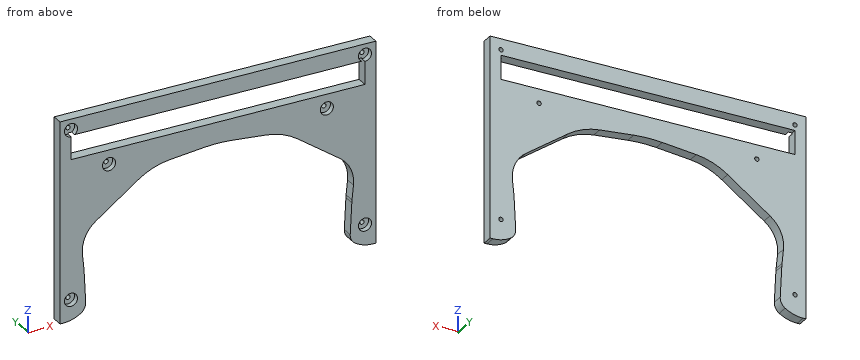
```python
from build123d import *

# Parameters (mm, degrees)
BOSS_EXTRU_1_DEPTH       = 10
ESQUISSE3_R              = 2
ENL_V_MAT_EXTRU_1_DEPTH  = 10
ESQUISSE6_W              = 270
ESQUISSE6_H              = 22
ENL_V_MAT_EXTRU_4_DEPTH  = 10
ESQUISSE9_R              = 2
ENL_V_MAT_EXTRU_7_DEPTH  = 10
ENL_V_MAT_EXTRU_9_DEPTH  = 10
CONG_5_R                 = 10
ESQUISSE12_R             = 2
ENL_V_MAT_EXTRU_10_DEPTH = 10
ESQUISSE14_R             = 6
ENL_V_MAT_EXTRU_11_DEPTH = 5


with BuildPart() as part:
    # Esquisse2 → Boss.-Extru.1 (new body)
    with BuildSketch(Plane(origin=(0, 0, 0), x_dir=(1, 0, 0), z_dir=(0, 1, 0))):
        with BuildLine():
            Line((0, 0), (290, 0))
            Line((290, 0), (290, 184.53))
            Line((290, 184.53), (287.426406871, 184.53))
            ThreePointArc((287.426406871, 184.53), (275.9459039, 182.246385975), (266.213203436, 175.743203436))
            Line((266.213203436, 175.743203436), (180.47, 90))
            Line((180.47, 90), (109.53, 90))
            Line((109.53, 90), (23.786796564, 175.743203436))
            ThreePointArc((23.786796564, 175.743203436), (14.0540961, 182.246385975), (2.573593129, 184.53))
            Line((2.573593129, 184.53), (0, 184.53))
            Line((0, 184.53), (0, 0))
        make_face()
    extrude(amount=BOSS_EXTRU_1_DEPTH)

    # Esquisse3 → Enlèv. mat.-Extru.1 (cut)
    with BuildSketch(Plane(origin=(0, 10, 0), x_dir=(1, 0, 0), z_dir=(0, 1, 0))):
        with Locations((10, 10)):
            Circle(ESQUISSE3_R)
        with Locations((280, 10)):
            Circle(ESQUISSE3_R)
    extrude(amount=-ENL_V_MAT_EXTRU_1_DEPTH, mode=Mode.SUBTRACT)

    # Esquisse6 → Enlèv. mat.-Extru.4 (cut)
    with BuildSketch(Plane(origin=(0, 10, 0), x_dir=(1, 0, 0), z_dir=(0, 1, 0))):
        with Locations((145, 26)):
            Rectangle(ESQUISSE6_W, ESQUISSE6_H)
    extrude(amount=-ENL_V_MAT_EXTRU_4_DEPTH, mode=Mode.SUBTRACT)

    # Esquisse9 → Enlèv. mat.-Extru.7 (cut)
    with BuildSketch(Plane(origin=(0, 10, 0), x_dir=(1, 0, 0), z_dir=(0, 1, 0))):
        with Locations((45, 50)):
            Circle(ESQUISSE9_R)
        with Locations((245, 50)):
            Circle(ESQUISSE9_R)
    extrude(amount=-ENL_V_MAT_EXTRU_7_DEPTH, mode=Mode.SUBTRACT)

    # Esquisse11 → Enlèv. mat.-Extru.9 (cut)
    with BuildSketch(Plane.XZ):
        with BuildLine():
            Line((23.786796564, -175.743203436), (22.069258887, -141.969600166))
            ThreePointArc((22.069258887, -141.969600166), (21.990433689, -140.725538115), (21.88061952, -139.483827743))
            Line((21.88061952, -139.483827743), (20.54302042, -126.242335439))
            ThreePointArc((20.54302042, -126.242335439), (23.053468491, -110.871931551), (32.931464028, -98.831297457))
            Line((32.931464028, -98.831297457), (71.774958897, -71.031800705))
            ThreePointArc((71.774958897, -71.031800705), (85.505992048, -63.689345624), (100.664013996, -60.127423581))
            Line((100.664013996, -60.127423581), (131.934446663, -56.968617789))
            ThreePointArc((131.934446663, -56.968617789), (145, -56.310379475), (158.065553337, -56.968617789))
            Line((158.065553337, -56.968617789), (189.335986004, -60.127423581))
            ThreePointArc((189.335986004, -60.127423581), (204.494007952, -63.689345624), (218.225041103, -71.031800705))
            Line((218.225041103, -71.031800705), (257.068535972, -98.831297457))
            ThreePointArc((257.068535972, -98.831297457), (266.946531509, -110.871931551), (269.45697958, -126.242335439))
            Line((269.45697958, -126.242335439), (268.11938048, -139.483827743))
            ThreePointArc((268.11938048, -139.483827743), (268.009566311, -140.725538115), (267.930741113, -141.969600166))
            Line((267.930741113, -141.969600166), (266.213203436, -175.743203436))
            Line((266.213203436, -175.743203436), (23.786796564, -175.743203436))
        make_face()
    extrude(amount=-ENL_V_MAT_EXTRU_9_DEPTH, mode=Mode.SUBTRACT)

    # Congé5
    cong_5_edges = [part.edges().sort_by_distance(p)[0] for p in [
        (23.786796564, 5, -175.743203436),
        (266.213203436, 5, -175.743203436),
    ]]
    fillet(cong_5_edges, radius=CONG_5_R)

    # Esquisse12 → Enlèv. mat.-Extru.10 (cut)
    with BuildSketch(Plane.XZ):
        with Locations((10, -165)):
            Circle(ESQUISSE12_R)
        with Locations((280, -165)):
            Circle(ESQUISSE12_R)
    extrude(amount=-ENL_V_MAT_EXTRU_10_DEPTH, mode=Mode.SUBTRACT)

    # Esquisse14 → Enlèv. mat.-Extru.11 (cut)
    with BuildSketch(Plane.XZ):
        with Locations((10, -10)):
            Circle(ESQUISSE14_R)
        with Locations((45, -50)):
            Circle(ESQUISSE14_R)
        with Locations((10, -165)):
            Circle(ESQUISSE14_R)
        with Locations((280, -165)):
            Circle(ESQUISSE14_R)
        with Locations((245, -50)):
            Circle(ESQUISSE14_R)
        with Locations((280, -10)):
            Circle(ESQUISSE14_R)
    extrude(amount=-ENL_V_MAT_EXTRU_11_DEPTH, mode=Mode.SUBTRACT)


solid = part.part
```
Input: part model. Units: mm. Frame: model coordinates. Coordinates: 2 decimals unless noted, no trailing zeros. Loops run counter-clockwise (first coordinate to the right, second up) from the corner with the lowest first, then second, coordinate; pieces in that order, holes last. Notation, with made-up numbers: (10.5, 17.25) -> (31.5, 17.25) arc R11 cw to (31.5, 22.25) -> close; hole circle Ø6 at (68, 45.5). An arc over 180 degrees is marked (long way). Use a Markdown table: item, result.
1) Cut plane C-C (y = 8.25). Give the number of separate pieces and of enclosed holes in the cut face, then the cut area to 3 significant figures.
Results found:
| item | result |
|---|---|
| separate pieces | 1 |
| enclosed holes | 7 |
| area | 19,800 mm2 |
2) Cut plane B-B (z = -82). Return the cut outline in (x, y), then the cut area to 3 significant figures.
Results found:
| item | result |
|---|---|
| outline | (0, 0) -> (56.45, 0) -> (56.45, 10) -> (0, 10) -> close; (233.55, 0) -> (290, 0) -> (290, 10) -> (233.55, 10) -> close |
| area | 1,130 mm2 |
3) Cut plane A-A (x = 67). Return the cut outline in (y, z), then the cut area to 3 significant figures.
Results found:
| item | result |
|---|---|
| outline | (0, -74.45) -> (10, -74.45) -> (10, -37) -> (0, -37) -> close; (0, -15) -> (10, -15) -> (10, 0) -> (0, 0) -> close |
| area | 524 mm2 |
4) Contact query for flat-ended pins moving along their axis: pin 1 (3.5 mm diameter, centred on x = 279.5, z = -166, fed in from -Y); pin 2 (6 mm diameter, centred on x = 187, y = 5.5, fed in from -Z); pin 3 (3 mm diameter, centred on x = 75.5, y = 3, fed in from -Z). Output: stop coordinate, or through.
Results found:
| item | result |
|---|---|
| pin 1 | stops at y = 5 |
| pin 2 | stops at z = -60.2 |
| pin 3 | stops at z = -69.51 |
5) Material intervals for line 1 along X through (y, z) = (3.4, -10); line 2 along X through (y, z) = (6.7, -50); line 3 along X through (y, z) = (4.75, -126), sorted ascending. Write a range as from..to.
Results found:
| item | result |
|---|---|
| line 1 | x = 0..4, 16..274, 286..290 |
| line 2 | x = 0..43, 47..243, 247..290 |
| line 3 | x = 0..20.52, 269.48..290 |
